Could you check a few things on this model? Use its own coordinates, in mm. A direction names the side the tool comes from. Coordinates: 2 decimals unless noted, no trailing zeros. Write each loop counter-clockwise with the first axis right and the second up, starting at its lowest first coordinate (ties: lowest second). Pieces come first, ordered by that corner, then holes.
```python
from build123d import *

# Parameters (mm, degrees)
SKETCH1_W           = 15
SKETCH1_H           = 27
SKETCH1_R           = 2
BOSS_EXTRUDE1_DEPTH = 5
SKETCH2_W           = 4
SKETCH2_H           = 10.5
BOSS_EXTRUDE2_DEPTH = 27
SKETCH4_R           = 0.75
CUT_EXTRUDE1_DEPTH  = 54


with BuildPart() as part:
    # Sketch1 → Boss-Extrude1 (new body)
    with BuildSketch(Plane(origin=(0, 0, 0), x_dir=(1, 0, 0), z_dir=(0, 1, 0))):
        with Locations((7.5, 13.5)):
            Rectangle(SKETCH1_W, SKETCH1_H)
        with Locations((8, 10)):
            Circle(SKETCH1_R, mode=Mode.SUBTRACT)
        with Locations((8, 20)):
            Circle(SKETCH1_R, mode=Mode.SUBTRACT)
    extrude(amount=BOSS_EXTRUDE1_DEPTH)

    # Sketch2 → Boss-Extrude2 (add)
    with BuildSketch(Plane.XY):
        with Locations((-2, -0.25)):
            Rectangle(SKETCH2_W, SKETCH2_H)
    extrude(amount=-BOSS_EXTRUDE2_DEPTH)

    # Mirror3: part across plane


with BuildPart() as part_1:
    add(part.part)
    add(part.part.mirror(Plane(origin=(0, -2.75, 0), x_dir=(0, 0, 1), z_dir=(0, -1, 0))))

    # Mirror4: part across plane


with BuildPart() as part_2:
    add(part_1.part)
    add(part_1.part.mirror(Plane(origin=(0, 5, 0), x_dir=(1, 0, 0), z_dir=(0, 0, -1))))

    # Sketch4 → Cut-Extrude1 (cut)
    with BuildSketch(Plane.XY.offset(27)):
        Circle(SKETCH4_R)
        with Locations((0, -5.5)):
            Circle(SKETCH4_R)
    extrude(amount=-CUT_EXTRUDE1_DEPTH, mode=Mode.SUBTRACT)


solid = part_2.part
```
Item 1: If I drill on line 1 along Z through (x, y) = (8, -7.6); line 2 along Y through (x, z) = (13.25, 14); line 3 along Z through (x, y) = (6.75, -9.25), over which ranges is the centre line in solid material (lowest first)?
Item 2: Which directions (+Z, -Z, +X, -X, +Y, -Y) give clear straight access to the entire face, cutting with the end or side of a thin tool? Please do faces 1 (the cylindrical face through (-0.51, 0.55, 0.38)), 2 (the flat face through (8, 0, 0)).
Item 3: If we mould it in two halves opening along X, with no side actions, what happens to faces 3 (the flat face through (0, -3, 0)), 4 (the cylindrical face through (8, -8, 22)), 5 (the flat face through (8, -5.5, 0))? For each: released by +X, released by -X, zero draft, split by the parting line, or undercut.
Item 4: Will these pins go through, and if not, where does the flat tip stop? pin 1 Ø1.2 at (y, z) = (-3, -8) entering from +X; pin 2 Ø2.5 at (x, z) = (8, 20) entering from +Y.
Item 5: I want a section at C-C, the plane y = -9.25. List the corners of the cut face in (x, z) for me, then the cut area to 3 significant figures.
Item 6: I want a section at A-A, the plane x = 12. List the corners of the cut face in (y, z) for me.
Item 7: I want a section at B-B, the plane z = -10. List the corners of the cut face in (x, y) for me.
Item 8: I want a section at D-D, the plane x = 8. Count the separate pieces of the cut face and the enclosed holes in it, then the cut area to 3 significant figures.
Taken from the geometry:
1. line 1: z = -27 to -22, -18 to -12, -8 to 8, 12 to 18, 22 to 27
1. line 2: y = -10.5 to -5.5, 0 to 5
1. line 3: z = -27 to -21.56, -18.44 to -11.56, -8.44 to 8.44, 11.56 to 18.44, 21.56 to 27
2. face 1: +Z, -Z
2. face 2: +Z, -Z, +X
3. face 3: released by +X
3. face 4: undercut
3. face 5: zero draft
4. pin 1: stops at x = 0
4. pin 2: passes through
5. outline: (-4, -27) - (15, -27) - (15, 27) - (-4, 27) - close; hole circle Ø4 at (8, -20); hole circle Ø4 at (8, -10); hole circle Ø4 at (8, 10); hole circle Ø4 at (8, 20)
5. area: 976 mm2
6. outline: (-10.5, -27) - (-5.5, -27) - (-5.5, 27) - (-10.5, 27) - close; (0, -27) - (5, -27) - (5, 27) - (0, 27) - close
7. outline: (-4, -10.5) - (6, -10.5) - (6, -5.5) - (0.75, -5.5) arc R0.75 cw (long way) to (0, -4.75) - (0, -0.75) arc R0.75 cw (long way) to (0.75, 0) - (6, 0) - (6, 5) - (-4, 5) - close; (10, -10.5) - (15, -10.5) - (15, -5.5) - (10, -5.5) - close; (10, 0) - (15, 0) - (15, 5) - (10, 5) - close
8. separate pieces: 10
8. enclosed holes: 0
8. area: 380 mm2
